For this review, take the finished solid that the model builds, in its own axes (mm). Round coordinates to 2 decimals unless told otherwise and drop trailing zeros. Loops run counter-clockwise (first coordinate to the right, second up) from the corner with the lowest first, then second, coordinate; pieces in that order, holes last.
1. Consider section A-A on x = 8.25. State the section outline as (y, z) points, then the cut area to 3 significant figures.
2. Consider section B-B on y = -26.75. State the section outline as (x, z) points, then the cut area to 3 significant figures.
3. To check wall thickness, follow line 1 along Y through (x, z) = (0, 3.75); line 2 along X through (y, z) = (-2, 0.55); line 3 along X through (y, z) = (-11, 1.2). State the ranges of each line that lie inside material, in increasing order.
4. Clearance check with flat-ended pins moving along their axes: pin 1 Ø0.8 at (x, y) = (23.5, 13) entering from -Z; pin 2 Ø1.5 at (x, z) = (-19, 1.5) entering from -Y. State where each tip first meets the part, or that it passes through.
5. Consider section C-C on x = -7.5. State how many separate pieces and enclosed holes the cut face has, then the cut area to 3 significant figures.
from build123d import *

# Parameters (mm, degrees)
SKETCH1_R                               = 31.75
ELBOW_PLATE_DEPTH                       = 4
SKETCH3_R                               = 1.33
SCREW_HOLES_DEPTH                       = 3
CABLE_SLOT_DEPTH                        = 4
FILLET1_R                               = 2
CBORE_FOR_M6_HEX_HEAD_BOLT1_D           = 4
CBORE_FOR_M6_HEX_HEAD_BOLT1_CBORE_D     = 7.5
CBORE_FOR_M6_HEX_HEAD_BOLT1_CBORE_DEPTH = 2.5


with BuildPart() as part:
    # Sketch1 → Elbow Plate (new body)
    with BuildSketch(Plane.XY):
        Circle(SKETCH1_R)
    extrude(amount=ELBOW_PLATE_DEPTH)

    # Sketch3 → Screw Holes (cut)
    with BuildSketch(Plane(origin=(0, 0, 0), x_dir=(-1, 0, 0), z_dir=(0, 0, -1))):
        with Locations((0, 26.75)):
            Circle(SKETCH3_R)
        with Locations((23.166179551, 13.375)):
            Circle(SKETCH3_R)
        with Locations((23.166179551, -13.375)):
            Circle(SKETCH3_R)
        with Locations((0, -26.75)):
            Circle(SKETCH3_R)
        with Locations((-23.166179551, -13.375)):
            Circle(SKETCH3_R)
        with Locations((-23.166179551, 13.375)):
            Circle(SKETCH3_R)
    extrude(amount=-SCREW_HOLES_DEPTH, mode=Mode.SUBTRACT)

    # Sketch4 → Cable Slot (cut)
    with BuildSketch(Plane.XY.offset(4)):
        with BuildLine():
            ThreePointArc((0, -23.172318516), (5.001159258, -18.171159258), (0, -13.17))
            ThreePointArc((0, -13.17), (-13.17, 0), (0, 13.17))
            ThreePointArc((0, 13.17), (5.001159258, 18.171159258), (0, 23.172318516))
            ThreePointArc((0, 23.172318516), (-23.172318516, 0), (0, -23.172318516))
        make_face()
    extrude(amount=-CABLE_SLOT_DEPTH, mode=Mode.SUBTRACT)

    # Fillet1
    fillet1_edges = [part.edges().sort_by_distance(p)[0] for p in [
        (-23.172318516, 0, 0),
        (5.001159258, 18.171159258, 0),
        (-13.17, 0, 0),
        (5.001159258, -18.171159258, 0),
    ]]
    fillet(fillet1_edges, radius=FILLET1_R)

    # CBORE for M6 Hex Head Bolt1 (through all)
    with Locations(Plane(origin=(0, 0, 0), x_dir=(-1, 0, 0), z_dir=(0, 0, -1))):
        with Locations((-8.25, 0), (0, -8.25), (8.25, 0), (0, 8.25)):
            CounterBoreHole(CBORE_FOR_M6_HEX_HEAD_BOLT1_D / 2, CBORE_FOR_M6_HEX_HEAD_BOLT1_CBORE_D / 2, CBORE_FOR_M6_HEX_HEAD_BOLT1_CBORE_DEPTH)


solid = part.part
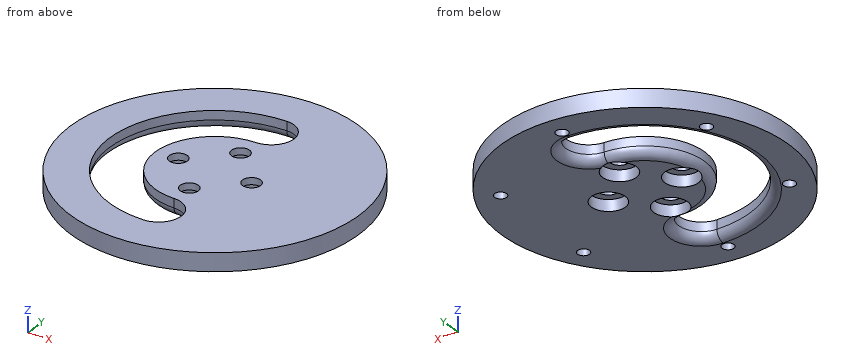
Resolved:
1. outline: (-30.66, 0) - (-3.75, 0) - (-3.75, 2.5) - (-2, 2.5) - (-2, 4) - (-30.66, 4) - close; (2, 2.5) - (3.75, 2.5) - (3.75, 0) - (30.66, 0) - (30.66, 4) - (2, 4) - close
1. area: 221 mm2
2. outline: (-17.1, 0) - (-1.33, 0) - (-1.33, 3) - (1.33, 3) - (1.33, 0) - (17.1, 0) - (17.1, 4) - (-17.1, 4) - close
2. area: 129 mm2
3. line 1: y = -31.75 to -23.17, -13.17 to -10.25, -6.25 to 6.25, 10.25 to 13.17, 23.17 to 31.75
3. line 2: x = -31.69 to -23.71, -12.39 to -11.42, -5.08 to 5.08, 11.42 to 31.69
3. line 3: x = -29.78 to -20.58, -6.93 to -2.55, 2.55 to 29.78
4. pin 1: stops at z = 3
4. pin 2: stops at y = -25.98
5. separate pieces: 4
5. enclosed holes: 0
5. area: 130 mm2
